from build123d import *

# Parameters (mm, degrees)
BOSS_EXTRUDE1_DEPTH = 19
SKETCH4_R           = 2.55
CUT_EXTRUDE1_DEPTH  = 139.686697271
LPATTERN1_COUNT     = 4
LPATTERN1_PITCH     = 8.3
FILLET2_R           = 5
BOSS_EXTRUDE4_DEPTH = 19
BOSS_EXTRUDE5_DEPTH = 2
LPATTERN3_COUNT     = 3
LPATTERN3_PITCH     = 8.5
FILLET4_R           = 20
SKETCH9_R           = 2.15
BOSS_EXTRUDE6_DEPTH = 19
FILLET5_R           = 5


with BuildPart() as part:
    # Sketch1 → Boss-Extrude1 (new body)
    with BuildSketch(Plane(origin=(0, 0, 0), x_dir=(1, 0, 0), z_dir=(0, 1, 0))):
        with BuildLine():
            Line((0, 0), (90, 0))
            ThreePointArc((90, 0), (109.091883092, -7.908116908), (117, -27))
            Line((117, -27), (117, -72))
            Line((117, -72), (110, -72))
            Line((110, -72), (110, -27))
            ThreePointArc((110, -27), (104.142135624, -12.857864376), (90, -7))
            Line((90, -7), (0, -7))
            Line((0, -7), (0, 0))
        make_face()
    extrude(amount=BOSS_EXTRUDE1_DEPTH)

    # Sketch4 → Cut-Extrude1 (cut, through all)
    with BuildSketch(Plane(origin=(0, 0, 0), x_dir=(0, 0, -1), z_dir=(1, 0, 0))):
        with Locations(Location((-64.5, 9.5, 0), (0, 0, 180))):
            Circle(SKETCH4_R)
    cut_extrude1 = extrude(amount=CUT_EXTRUDE1_DEPTH, mode=Mode.SUBTRACT)

    # LPattern1: Cut-Extrude1 ×4
    with Locations(*[(0, 0, -i * LPATTERN1_PITCH) for i in range(1, LPATTERN1_COUNT)]):
        add(cut_extrude1, mode=Mode.SUBTRACT)

    # Fillet2
    fillet2_edges = [part.edges().sort_by_distance(p)[0] for p in [
        (0, 0, 3.5),
        (113.5, 19, 72),
        (0, 19, 3.5),
        (113.5, 0, 72),
    ]]
    fillet(fillet2_edges, radius=FILLET2_R)

    # Sketch6 → Boss-Extrude4 (add)
    with BuildSketch(Plane(origin=(0, 0, 0), x_dir=(1, 0, 0), z_dir=(0, 1, 0))):
        with BuildLine():
            Line((57.067989457, 0), (96.460545107, 3))
            ThreePointArc((96.460545107, 3), (115.383129249, -6.075834674), (117, -27))
            ThreePointArc((117, -27), (109.091883092, -7.908116908), (90, 0))
            Line((90, 0), (57.067989457, 0))
        make_face()
    extrude(amount=BOSS_EXTRUDE4_DEPTH)

    # Sketch8 → Boss-Extrude5 (add)
    with BuildSketch(Plane(origin=(0, 0, 0), x_dir=(1, 0, 0), z_dir=(0, 1, 0))):
        with BuildLine():
            ThreePointArc((90, -7), (102.578584062, -14.421415938), (110, -27))
            ThreePointArc((110, -27), (104.142135624, -12.857864376), (90, -7))
        make_face()
    boss_extrude5 = extrude(amount=BOSS_EXTRUDE5_DEPTH)

    # LPattern3: Boss-Extrude5 ×3
    with Locations(*[(0, i * LPATTERN3_PITCH, 0) for i in range(1, LPATTERN3_COUNT)]):
        add(boss_extrude5)

    # Fillet4
    # the kernel refuses this fillet: 20 mm, written as the material it adds along each edge
    with BuildSketch(Plane(origin=(57.067989457, 0, 0), x_dir=(-1, 0, 0), z_dir=(0, 1, 0))) as fillet4_piece_1:
        with BuildLine():
            CenterArc((FILLET4_R * 0.0380232084134, -FILLET4_R), FILLET4_R, 90, 4.355040752)
            Line((-FILLET4_R * 0.0379134219382, -FILLET4_R * 0.00288735432207), (0, 0))
            Line((0, 0), (FILLET4_R * 0.0380232084134, 0))
        make_face()
    extrude(amount=19)

    # Sketch9 → Boss-Extrude6 (add)
    with BuildSketch(Plane.ZY.offset(-10)):
        with BuildLine():
            Line((7, 14), (12, 14))
            ThreePointArc((12, 14), (17, 9), (12, 4))
            Line((12, 4), (7, 4))
            Line((7, 4), (7, 14))
        make_face()
        with Locations((12, 9)):
            Circle(SKETCH9_R, mode=Mode.SUBTRACT)
    extrude(amount=-BOSS_EXTRUDE6_DEPTH)

    # Fillet5
    # the kernel refuses this fillet: 5 mm, written as the material it adds along each edge
    with BuildSketch(Plane(origin=(10, 4, 7), x_dir=(0, -1.0, 1.5822898546952626e-12), z_dir=(1, 0, 0))) as fillet5_piece_1:
        with BuildLine():
            CenterArc((5, -4.898979486), FILLET5_R, 101.536959033, 78.463040967)
            Line((0, -4.898979486), (0, 0))
            Line((0, 0), (4, 0))
        make_face()
    extrude(amount=19)
    with BuildSketch(Plane(origin=(10, 14, 7), x_dir=(0, 1, 0), z_dir=(1, 0, 0))) as fillet5_piece_2:
        with BuildLine():
            CenterArc((FILLET5_R, FILLET5_R), FILLET5_R, 180, 90)
            Line((0, FILLET5_R), (0, 0))
            Line((0, 0), (FILLET5_R, 0))
        make_face()
    extrude(amount=19)


solid = part.part
The model under review builds one solid part; all positions refer to its coordinate system, in mm. A direction names the side the tool comes from. Coordinates: 2 decimals unless noted, no trailing zeros. Loops run counter-clockwise (first coordinate to the right, second up) from the corner with the lowest first, then second, coordinate; pieces in that order, holes last. Notation, with made-up numbers: M 27,46 L 47,46 A21 ccw 47,74 Z; hole C 83,33.5 d2. An arc over 180 degrees is marked long. Put each result on its own line as item: value. Start each with the question number.
Q1. Wall thickness on line 1 (Y direction, x = 25, z = 12); line 2 (Y direction, x = 115, z = 64); line 3 (X direction, y = 1.5, z = 49): over which ranges is each line inside the solid? List them lowest first.
Q2. Add section C-C (y = 15.75). Write out the cut boundary in (x, z), and give its area (3 significant figures).
Q3. Add section B-B (x = 111.5). Write out the cut boundary in (y, z), and give its area (3 significant figures).
Q4. The part is to be moulded in two halves that separate along X. For faces 4 (the flat face through (10, 7.5, 9.8)), 5 (the flat face through (83, 0, 6)), 6 (the flat face through (103, 8.5, 14)), say which applies: +X half, -X half, draft (parallel to the pull), parting line (faces both ways), or undercut.
Q5. Clearance check with flat-ended pins moving along their axes: pin 1 (9.5 mm diameter, centred on x = 71, y = 12, fed in from +Z); pin 2 (3 mm diameter, centred on y = 9.5, z = 6, fed in from +X); pin 3 (3 mm diameter, centred on y = 14.5, z = 41.5, fed in from -X). State where each tip first meets the part, or that it passes through.
Q6. Add section D-D (x = 93.5). Write out the cut boundary in (y, z), and give its area (3 significant figures).
Q7. For faces 1 (the cylindrical face through (104.297, 13.704, 13.014)), 2 (the flat face through (28, 9, 0)), 3 (the cylindrical face through (19.37, 10.81, 13.16)), list the 3-axis set-ups (+Z, -Z, +X, -X, +Y, -Y) from which the entire face can be reached by the end or side of a thin tool; tool diameter is ignored.
Q8. Add section A-A (z = 56.2). Write out the cut boundary in (x, y), and give its area (3 significant figures).
Answers:
1. line 1: y = 4 to 6.85, 11.15 to 14
1. line 2: y = 0 to 7, 12 to 19
1. line 3: x = 110 to 117
2. outline: M 0.32,0 L 56.31,0 A20 cw 57.83,-0.06 L 96.46,-3 A21 ccw 117,27 L 117,71.68 L 110,71.68 L 110,27 A20 cw 90,7 L 29,7 L 29,8.2 L 10,8.2 L 10,7 L 0.32,7 Z
2. area: 1,460 mm^2
3. outline: M 0,1.81 L 19,1.81 L 19,67 A5 ccw 14,72 L 5,72 A5 ccw 0,67 Z; hole C 9.5,39.6 d5.1; hole C 9.5,47.9 d5.1; hole C 9.5,56.2 d5.1; hole C 9.5,64.5 d5.1
3. area: 1,240 mm^2
4. face 4: -X half
4. face 5: draft
4. face 6: undercut
5. pin 1: stops at z = 7
5. pin 2: stops at x = 116.28
5. pin 3: stops at x = 110
6. outline: M 0,-2.77 L 19,-2.77 L 19,8.25 L 17,8.25 L 17,7.31 L 10.5,7.31 L 10.5,8.25 L 8.5,8.25 L 8.5,7.31 L 2,7.31 L 2,8.25 L 0,8.25 Z
6. area: 197 mm^2
7. face 1: +Z
7. face 2: -Z, -X, +Y, -Y
7. face 3: -X
8. outline: M 110,0 L 117,0 L 117,6.95 L 110,6.95 Z; M 110,12.05 L 117,12.05 L 117,19 L 110,19 Z
8. area: 97.3 mm^2
